Check sheet for the modelled part. Datum: model origin and axes. Units: mm. Coordinates: 2 decimals unless noted, no trailing zeros. Loops run counter-clockwise (first coordinate to the right, second up) from the corner with the lowest first, then second, coordinate; pieces in that order, holes last. Notation, with made-up numbers: M 59.5,28.25 L 87.5,28.25 A35 ccw 87.5,62.25 Z; hole C -21,39 d2. An arc over 180 degrees is marked long. Return JSON: item names as keys, results as strings.
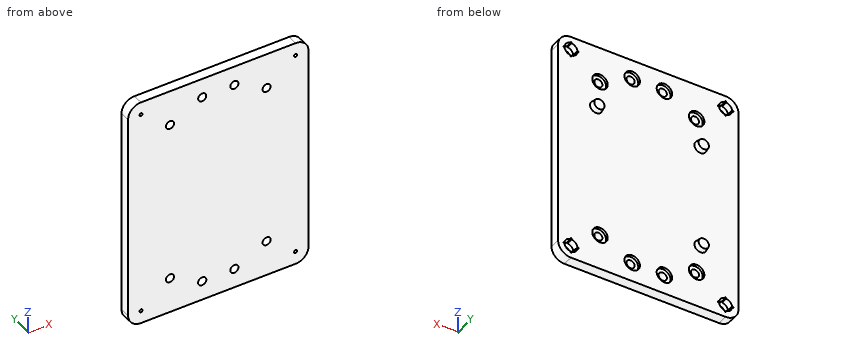
from build123d import *

# Parameters (mm, degrees)
SKETCH_1_W                                 = 200
SKETCH_1_H                                 = 200
SKETCH_1_R                                 = 3.2
SKETCH_1_R_2                               = 3.15
EXTRUDE_1_DEPTH                            = 8
SKETCH_2_R                                 = 6
CUT_EXTRUDE_1_DEPTH                        = 2
SKETCH_3_W                                 = 200
SKETCH_3_H                                 = 200
SKETCH_3_W_2                               = 140
SKETCH_3_H_2                               = 180
CUT_EXTRUDE_2_DEPTH                        = 10
FILLET_1_R                                 = 10
FILLET_2_R                                 = 10
FILLET_3_R                                 = 10
FILLET_4_R                                 = 10
CUT_EXTRUDE_5_DEPTH                        = 5
MIRROR_7_AT_THE_SECOND_PLANE_COPY_1_DEPTH  = 5
SKETCH_15_R                                = 4
EXTRUDE_2_DEPTH                            = 4
DRAFT_3_ANGLE                              = 10
DRAFT_3_OF_MIRROR_13_2_ANGLE               = 10
DRAFT_3_OF_MIRROR_14_2_ANGLE               = 10
SKETCH_16_R                                = 1.2
CUT_EXTRUDE_6_DEPTH                        = 115.297856498
MIRROR_15_AT_THE_SECOND_PLANE_COPY_1_SKE_R = 1.2
MIRROR_15_AT_THE_SECOND_PLANE_COPY_1_DEPTH = 115.297856498


with BuildPart() as part:
    # 草图1 → 凸台-拉伸1 (new body)
    with BuildSketch(Plane(origin=(0, 0, 0), x_dir=(1, 0, 0), z_dir=(0, 1, 0))):
        Rectangle(SKETCH_1_W, SKETCH_1_H)
        with Locations(Location((-12.5, 75, 0), (0, 0, 270))):
            Circle(SKETCH_1_R, mode=Mode.SUBTRACT)
        with Locations(Location((12.5, 75, 0), (0, 0, 270))):
            Circle(SKETCH_1_R_2, mode=Mode.SUBTRACT)
        with Locations(Location((-12.5, -75, 0), (0, 0, 270))):
            Circle(SKETCH_1_R_2, mode=Mode.SUBTRACT)
        with Locations(Location((12.5, -75, 0), (0, 0, 270))):
            Circle(SKETCH_1_R_2, mode=Mode.SUBTRACT)
        with Locations(Location((-37.5, -62.5, 0), (0, 0, 270))):
            Circle(SKETCH_1_R_2, mode=Mode.SUBTRACT)
        with Locations(Location((37.5, -62.5, 0), (0, 0, 270))):
            Circle(SKETCH_1_R_2, mode=Mode.SUBTRACT)
        with Locations(Location((-37.5, 62.5, 0), (0, 0, 270))):
            Circle(SKETCH_1_R_2, mode=Mode.SUBTRACT)
        with Locations(Location((37.5, 62.5, 0), (0, 0, 270))):
            Circle(SKETCH_1_R_2, mode=Mode.SUBTRACT)
    extrude(amount=EXTRUDE_1_DEPTH)

    # 草图2 → 切除-拉伸1 (cut)
    with BuildSketch(Plane(origin=(0, 8, 0), x_dir=(1, 0, 0), z_dir=(0, 1, 0))):
        with Locations(Location((-37.5, 62.5, 0), (0, 0, 270))):
            Circle(SKETCH_2_R)
        with Locations(Location((-12.5, 75, 0), (0, 0, 270))):
            Circle(SKETCH_2_R)
        with Locations(Location((12.5, 75, 0), (0, 0, 270))):
            Circle(SKETCH_2_R)
        with Locations(Location((37.5, 62.5, 0), (0, 0, 270))):
            Circle(SKETCH_2_R)
        with Locations(Location((-37.5, -62.5, 0), (0, 0, 270))):
            Circle(SKETCH_2_R)
        with Locations(Location((-12.5, -75, 0), (0, 0, 270))):
            Circle(SKETCH_2_R)
        with Locations(Location((12.5, -75, 0), (0, 0, 270))):
            Circle(SKETCH_2_R)
        with Locations(Location((37.5, -62.5, 0), (0, 0, 270))):
            Circle(SKETCH_2_R)
    extrude(amount=-CUT_EXTRUDE_1_DEPTH, mode=Mode.SUBTRACT)

    # 草图3 → 切除-拉伸2 (cut)
    with BuildSketch(Plane(origin=(0, 8, 0), x_dir=(1, 0, 0), z_dir=(0, 1, 0))):
        Rectangle(SKETCH_3_W, SKETCH_3_H)
        Rectangle(SKETCH_3_W_2, SKETCH_3_H_2, mode=Mode.SUBTRACT)
    extrude(amount=-CUT_EXTRUDE_2_DEPTH, mode=Mode.SUBTRACT)

    # 圆角1
    fillet_1_edges = [part.edges().sort_by_distance(p)[0] for p in [
        (-70, 4, -90),
    ]]
    fillet(fillet_1_edges, radius=FILLET_1_R)

    # 圆角2
    fillet_2_edges = [part.edges().sort_by_distance(p)[0] for p in [
        (70, 4, -90),
    ]]
    fillet(fillet_2_edges, radius=FILLET_2_R)

    # 圆角3
    fillet_3_edges = [part.edges().sort_by_distance(p)[0] for p in [
        (70, 4, 90),
    ]]
    fillet(fillet_3_edges, radius=FILLET_3_R)

    # 圆角4
    fillet_4_edges = [part.edges().sort_by_distance(p)[0] for p in [
        (-70, 4, 90),
    ]]
    fillet(fillet_4_edges, radius=FILLET_4_R)

    # 草图12 → 切除-拉伸5 (cut)
    with BuildSketch(Plane(origin=(0, 8, 0), x_dir=(1, 0, 0), z_dir=(0, 1, 0))):
        with BuildLine():
            Line((-60.5, 84.974937186), (-60.5, 86))
            Line((-60.5, 86), (-59.5, 86))
            Line((-59.5, 86), (-59.5, 84.974937186))
            ThreePointArc((-59.5, 84.974937186), (-56.464466094, 83.535533906), (-55.025062814, 80.5))
            Line((-55.025062814, 80.5), (-54, 80.5))
            Line((-54, 80.5), (-54, 79.5))
            Line((-54, 79.5), (-55.025062814, 79.5))
            ThreePointArc((-55.025062814, 79.5), (-56.464466094, 76.464466094), (-59.5, 75.025062814))
            Line((-59.5, 75.025062814), (-59.5, 74))
            Line((-59.5, 74), (-60.5, 74))
            Line((-60.5, 74), (-60.5, 75.025062814))
            ThreePointArc((-60.5, 75.025062814), (-63.535533906, 76.464466094), (-64.974937186, 79.5))
            Line((-64.974937186, 79.5), (-66, 79.5))
            Line((-66, 79.5), (-66, 80.5))
            Line((-66, 80.5), (-64.974937186, 80.5))
            ThreePointArc((-64.974937186, 80.5), (-63.535533906, 83.535533906), (-60.5, 84.974937186))
        make_face()
    cut_extrude_5 = extrude(amount=-CUT_EXTRUDE_5_DEPTH, mode=Mode.SUBTRACT)

    # 镜向7: 切除-拉伸5 across plane
    add(cut_extrude_5.mirror(Plane.XY), mode=Mode.SUBTRACT)

    # 镜向7 at the second plane: 切除-拉伸5 across plane
    add(cut_extrude_5.mirror(Plane(origin=(0, 0, 0), x_dir=(0, 0, 1), z_dir=(1, 0, 0))), mode=Mode.SUBTRACT)

    # 镜向7 at the second plane copy 1 sket → 镜向7 at the second plane copy 1 (cut)
    with BuildSketch(Plane(origin=(0, 8, 0), x_dir=(-1, 0, 0), z_dir=(0, 1, 0))):
        with BuildLine():
            Line((-60.5, 84.974937186), (-60.5, 86))
            Line((-60.5, 86), (-59.5, 86))
            Line((-59.5, 86), (-59.5, 84.974937186))
            ThreePointArc((-59.5, 84.974937186), (-56.464466094, 83.535533906), (-55.025062814, 80.5))
            Line((-55.025062814, 80.5), (-54, 80.5))
            Line((-54, 80.5), (-54, 79.5))
            Line((-54, 79.5), (-55.025062814, 79.5))
            ThreePointArc((-55.025062814, 79.5), (-56.464466094, 76.464466094), (-59.5, 75.025062814))
            Line((-59.5, 75.025062814), (-59.5, 74))
            Line((-59.5, 74), (-60.5, 74))
            Line((-60.5, 74), (-60.5, 75.025062814))
            ThreePointArc((-60.5, 75.025062814), (-63.535533906, 76.464466094), (-64.974937186, 79.5))
            Line((-64.974937186, 79.5), (-66, 79.5))
            Line((-66, 79.5), (-66, 80.5))
            Line((-66, 80.5), (-64.974937186, 80.5))
            ThreePointArc((-64.974937186, 80.5), (-63.535533906, 83.535533906), (-60.5, 84.974937186))
        make_face()
    extrude(amount=-MIRROR_7_AT_THE_SECOND_PLANE_COPY_1_DEPTH, mode=Mode.SUBTRACT)

    # 草图15 → 凸台-拉伸2 (add)
    with BuildSketch(Plane(origin=(0, 8, 0), x_dir=(1, 0, 0), z_dir=(0, 1, 0))):
        with Locations(Location((-40.5, -40.5, 0), (0, 0, 270))):
            Circle(SKETCH_15_R)
    extrude_2 = extrude(amount=EXTRUDE_2_DEPTH)

    # 拔模3
    draft_3_faces = [part.faces().sort_by_distance(p)[0] for p in [
        (-40.5, 10, 36.5),
    ]]
    draft(draft_3_faces, Plane(origin=(-40.5, 12, 40.5), x_dir=(0, 0, 1), z_dir=(0, 1, 0)), DRAFT_3_ANGLE)

    # 镜向13: 凸台-拉伸2 across plane
    add(extrude_2.mirror(Plane.XY))

    # 拔模3 of Mirror 13 2
    draft_3_of_mirror_13_2_faces = [part.faces().sort_by_distance(p)[0] for p in [
        (-40.5, 10, -36.5),
    ]]
    draft(draft_3_of_mirror_13_2_faces, Plane(origin=(-40.5, 12, -40.5), x_dir=(0, 0, -1), z_dir=(0, 1, 0)), DRAFT_3_OF_MIRROR_13_2_ANGLE)

    # 镜向14: 凸台-拉伸2 across plane
    add(extrude_2.mirror(Plane(origin=(0, 0, 0), x_dir=(0, 0, 1), z_dir=(1, 0, 0))))

    # 拔模3 of Mirror 14 2
    draft_3_of_mirror_14_2_faces = [part.faces().sort_by_distance(p)[0] for p in [
        (40.5, 10, 36.5),
    ]]
    draft(draft_3_of_mirror_14_2_faces, Plane(origin=(40.5, 12, 40.5), x_dir=(0, 0, 1), z_dir=(0, 1, 0)), DRAFT_3_OF_MIRROR_14_2_ANGLE)

    # 草图16 → 切除-拉伸6 (cut, through all)
    with BuildSketch(Plane(origin=(0, 8, 0), x_dir=(1, 0, 0), z_dir=(0, 1, 0))):
        with Locations(Location((-60, 80, 0), (0, 0, 270))):
            Circle(SKETCH_16_R)
    cut_extrude_6 = extrude(amount=-CUT_EXTRUDE_6_DEPTH, mode=Mode.SUBTRACT)

    # 镜向15: 切除-拉伸6 across plane
    add(cut_extrude_6.mirror(Plane.XY), mode=Mode.SUBTRACT)

    # 镜向15 at the second plane: 切除-拉伸6 across plane
    add(cut_extrude_6.mirror(Plane(origin=(0, 0, 0), x_dir=(0, 0, 1), z_dir=(1, 0, 0))), mode=Mode.SUBTRACT)

    # 镜向15 at the second plane copy 1 ske → 镜向15 at the second plane copy 1 (cut, through all)
    with BuildSketch(Plane(origin=(0, 8, 0), x_dir=(-1, 0, 0), z_dir=(0, 1, 0))):
        with Locations(Location((-60, 80, 0), (0, 0, 270))):
            Circle(MIRROR_15_AT_THE_SECOND_PLANE_COPY_1_SKE_R)
    extrude(amount=-MIRROR_15_AT_THE_SECOND_PLANE_COPY_1_DEPTH, mode=Mode.SUBTRACT)


solid = part.part
1) Section check A-A on x = 12.5. Record the cut outline in (y, z).
Answers:
{"outline": "M 0,-90 L 8,-90 L 8,-81 L 6,-81 L 6,-78.15 L 0,-78.15 Z; M 0,-71.85 L 6,-71.85 L 6,-69 L 8,-69 L 8,69 L 6,69 L 6,71.85 L 0,71.85 Z; M 0,78.15 L 6,78.15 L 6,81 L 8,81 L 8,90 L 0,90 Z"}
2) Section check B-B on z = 40.5. Record the cut outline in (x, y).
Answers:
{"outline": "M -70,0 L 70,0 L 70,8 L 45.21,8 L 44.5,12 L 36.5,12 L 35.79,8 L -35.79,8 L -36.5,12 L -44.5,12 L -45.21,8 L -70,8 Z"}
3) Scan lines: line 1 along X through (y, z) = (7.05, -62.5); line 2 along X through (y, z) = (3.65, 62.5); line 3 along Z through (x, y) = (12.5, 4.2). Record each from-to range of solid material in increasing order. Write a range as [from, to].
Answers:
{"line 1": "[-70, -43.5], [-31.5, 31.5], [43.5, 70]", "line 2": "[-70, -40.65], [-34.35, 34.35], [40.65, 70]", "line 3": "[-90, -78.15], [-71.85, 71.85], [78.15, 90]"}
4) Section check C-C on x = -12.5. Record the cut outline in (y, z).
Answers:
{"outline": "M 0,-90 L 8,-90 L 8,-81 L 6,-81 L 6,-78.2 L 0,-78.2 Z; M 0,-71.8 L 6,-71.8 L 6,-69 L 8,-69 L 8,69 L 6,69 L 6,71.85 L 0,71.85 Z; M 0,78.15 L 6,78.15 L 6,81 L 8,81 L 8,90 L 0,90 Z"}
5) Section check D-D on y = 10. Record the cut outline in (x, z).
Answers:
{"outline": "C -40.5,-40.5 d8.71; C -40.5,40.5 d8.71; C 40.5,40.5 d8.71"}
6) Go/stop test with flat-tipped pins: pin 1 Ø6 at (x, z) = (-16.5, 5.5) entering from -Y; pin 2 Ø1.5 at (x, y) = (19, 9) entering from +Z; pin 3 Ø3 at (x, z) = (-33.5, 57) entering from +Y; pin 4 Ø4 at (x, z) = (60, 80) entering from +Y. Record where each tip stops, or that it passes through.
Answers:
{"pin 1": "y = 0", "pin 2": "through", "pin 3": "y = 8", "pin 4": "y = 3"}
